Source: CAD feature listing. Evaluate the final solid. Frame: model axes, mm. A direction names the side the tool comes from. Give positions to 0.01 mm unless a question says otherwise; leave off trailing zeros. Loops run counter-clockwise (first coordinate to the right, second up) from the corner with the lowest first, then second, coordinate; pieces in that order, holes last.
```python
from build123d import *

# Parameters (mm, degrees)
SKETCH_1_W          = 30
SKETCH_1_H          = 36
SKETCH_1_R          = 1.7
EXTRUDE_1_DEPTH     = 8
SKETCH_2_R          = 3.75
CUT_EXTRUDE_1_DEPTH = 4.5
SKETCH_3_W          = 15
SKETCH_3_H          = 20
SKETCH_3_R          = 4
EXTRUDE_4_DEPTH     = 8
SKETCH_8_W          = 10
SKETCH_8_H          = 40
EXTRUDE_5_DEPTH     = 30
SKETCH_10_W         = 12
SKETCH_10_H         = 12.5
SKETCH_10_W_2       = 5
CUT_EXTRUDE_4_DEPTH = 30
SKETCH_11_R         = 1.5
CUT_EXTRUDE_5_DEPTH = 47
SKETCH_12_W         = 2
SKETCH_12_H         = 25.842259392
SKETCH_12_H_2       = 30.756424204
CUT_EXTRUDE_6_DEPTH = 10
SKETCH_13_R         = 1.5
CUT_EXTRUDE_7_DEPTH = 40
SKETCH_14_W         = 5
SKETCH_14_H         = 12.5
CUT_EXTRUDE_8_DEPTH = 10


with BuildPart() as part:
    # 草图1 → 凸台-拉伸1 (new body)
    with BuildSketch(Plane.XY):
        with Locations((-3.375, -1.625)):
            Rectangle(SKETCH_1_W, SKETCH_1_H)
        with Locations((-12.375, 10.375)):
            Circle(SKETCH_1_R, mode=Mode.SUBTRACT)
        with Locations((-12.375, -13.625)):
            Circle(SKETCH_1_R, mode=Mode.SUBTRACT)
        with Locations(Location((5.625, -13.625, 0), (0, 0, 180))):
            Circle(SKETCH_1_R, mode=Mode.SUBTRACT)
        with Locations(Location((5.625, 10.375, 0), (0, 0, 180))):
            Circle(SKETCH_1_R, mode=Mode.SUBTRACT)
    extrude(amount=EXTRUDE_1_DEPTH)

    # 草图2 → 切除-拉伸1 (cut)
    with BuildSketch(Plane(origin=(0, 0, 0), x_dir=(-1, 0, 0), z_dir=(0, 0, -1))):
        with Locations((12.375, 10.375)):
            Circle(SKETCH_2_R)
        with Locations(Location((-5.625, 10.375, 0), (0, 0, 180))):
            Circle(SKETCH_2_R)
        with Locations(Location((12.375, -13.625, 0), (0, 0, 180))):
            Circle(SKETCH_2_R)
        with Locations((-5.625, -13.625)):
            Circle(SKETCH_2_R)
    extrude(amount=-CUT_EXTRUDE_1_DEPTH, mode=Mode.SUBTRACT)

    # 草图3 → 凸台-拉伸4 (add)
    # profile 1 of 2: a face of its own
    with BuildSketch(Plane.XY.offset(8)):
        with Locations((-10.875, 26.375)):
            Rectangle(SKETCH_3_W, SKETCH_3_H)
        with Locations((-10.875, 21.375)):
            Circle(SKETCH_3_R, mode=Mode.SUBTRACT)
    # profile 2 of 2: a face of its own
    with BuildSketch(Plane.XY.offset(8)):
        with Locations((-10.875, -29.625)):
            Rectangle(SKETCH_3_W, SKETCH_3_H)
        with Locations((-10.875, -24.625)):
            Circle(SKETCH_3_R, mode=Mode.SUBTRACT)
    extrude(amount=-EXTRUDE_4_DEPTH)

    # 草图8 → 凸台-拉伸5 (add)
    with BuildSketch(Plane.XY.offset(8)):
        with Locations((16.625, -1.625)):
            Rectangle(SKETCH_8_W, SKETCH_8_H)
    extrude(amount=-EXTRUDE_5_DEPTH)

    # 草图10 → 切除-拉伸4 (cut)
    with BuildSketch(Plane.ZY.offset(-11.625)):
        with Locations((-16, 7.125)):
            Rectangle(SKETCH_10_W, SKETCH_10_H)
        with Locations((-2.5, 7.125)):
            Rectangle(SKETCH_10_W_2, SKETCH_10_H)
        with Locations((-2.5, -10.375)):
            Rectangle(SKETCH_10_W_2, SKETCH_10_H)
        with Locations((-16, -10.375)):
            Rectangle(SKETCH_10_W, SKETCH_10_H)
    extrude(amount=-CUT_EXTRUDE_4_DEPTH, mode=Mode.SUBTRACT)

    # 草图11 → 切除-拉伸5 (cut)
    with BuildSketch(Plane(origin=(0, 18.375, 0), x_dir=(1, 0, 0), z_dir=(0, 1, 0))):
        with Locations(Location((16.621809271, 18.123313308, 0), (0, 0, 180))):
            Circle(SKETCH_11_R)
    extrude(amount=-CUT_EXTRUDE_5_DEPTH, mode=Mode.SUBTRACT)

    # 草图12 → 切除-拉伸6 (cut)
    with BuildSketch(Plane(origin=(0, 0, 0), x_dir=(-1, 0, 0), z_dir=(0, 0, -1))):
        with Locations((10.875, 36.375)):
            Rectangle(SKETCH_12_W, SKETCH_12_H)
        with Locations((10.875, -39.625)):
            Rectangle(SKETCH_12_W, SKETCH_12_H_2)
    extrude(amount=-CUT_EXTRUDE_6_DEPTH, mode=Mode.SUBTRACT)

    # 草图13 → 切除-拉伸7 (cut)
    with BuildSketch(Plane.ZY.offset(18.375)):
        with Locations((3.892451488, 31.868119268)):
            Circle(SKETCH_13_R)
        with Locations(Location((3.892451488, -35.118119268, 0), (0, 0, 270))):
            Circle(SKETCH_13_R)
    extrude(amount=-CUT_EXTRUDE_7_DEPTH, mode=Mode.SUBTRACT)

    # 草图14 → 切除-拉伸8 (cut)
    with BuildSketch(Plane(origin=(21.625, 0, 0), x_dir=(0, 0, -1), z_dir=(1, 0, 0))):
        with Locations((7.5, 7.125)):
            Rectangle(SKETCH_14_W, SKETCH_14_H)
        with Locations((7.5, -10.375)):
            Rectangle(SKETCH_14_W, SKETCH_14_H)
    extrude(amount=-CUT_EXTRUDE_8_DEPTH, mode=Mode.SUBTRACT)


solid = part.part
```
(1) Section A-A, the plane z = -12.5. Return the cut outline in (x, y) (3 decimals).
A:
outline: (11.625, -21.625) - (21.625, -21.625) - (21.625, -16.625) - (11.625, -16.625) - close; (11.625, -4.125) - (21.625, -4.125) - (21.625, 0.875) - (11.625, 0.875) - close; (11.625, 13.375) - (21.625, 13.375) - (21.625, 18.375) - (11.625, 18.375) - close
(2) Section C-C, the plane x = 14. Return the cut outline in (y, z) (3 decimals).
A:
outline: (-21.625, -22) - (-16.625, -22) - (-16.625, 0) - (-4.125, 0) - (-4.125, -22) - (0.875, -22) - (0.875, 0) - (13.375, 0) - (13.375, -22) - (18.375, -22) - (18.375, 8) - (-21.625, 8) - close
(3) Ray query, line 1 along Y through (x, z) = (18.5, -13.25) (3 decimals); line 2 along X through (y, z) = (12, 3.5) (3 decimals); line 3 along Y through (x, z) = (20, 2) (3 decimals). Return the intervals inside material, ascending.
A:
line 1: y = -21.625 to -16.625, -4.125 to 0.875, 13.375 to 18.375
line 2: x = -18.375 to -15.755, -8.995 to 2.245, 9.005 to 21.625
line 3: y = -21.625 to 18.375
(4) Reachability of faces 5 (the flat face through (-18.375, -2, 4)), 6 (the cylindrical face through (18.12, -19.09, -18.06)), 7 (the flat face through (17, 13.375, -11)), 8 (the flat face through (17, 18.375, -7)), 9 (the flat face through (-9.875, 29, 4)) from +Z, -Z, +X, -X, +Y, -Y: full face, straight path, thin tool, end or side. Return the list, or none.
A:
face 5: +Z, -Z, -X, +Y, -Y
face 6: +Y, -Y
face 7: -Z, +X, -X
face 8: +Z, -Z, +X, +Y
face 9: +Z, -Z, +Y
(5) First-contact query: pin 1 (2 mm diameter, centred on x = 4.5, y = -15, fed in from -Z); pin 2 (11 mm diameter, centred on x = 18.5, z = -15, fed in from +Y) (3 decimals); pin 3 (4 mm diameter, centred on y = -35, z = 2.5, fed in from +X) (3 decimals). Flat tips, straight axial feed; report the tip coordinate or a pass-through.
A:
pin 1: stops at z = 4.5
pin 2: stops at y = 18.375
pin 3: stops at x = -3.375
(6) Section B-B, the plane y = -32. Return the cut outline in (x, z) (3 decimals).
A:
outline: (-18.375, 0) - (-11.875, 0) - (-11.875, 8) - (-18.375, 8) - close; (-9.875, 0) - (-3.375, 0) - (-3.375, 8) - (-9.875, 8) - close
(7) Section D-D, the plane y = 0. Return the cut outline in (x, z) (3 decimals).
A:
outline: (-18.375, 0) - (11.625, 0) - (11.625, -22) - (21.625, -22) - (21.625, 8) - (-18.375, 8) - close; hole circle Ø3 at (16.622, -18.123)
(8) Mould query, pull axis Z, two halves, no side actions, for faces 1 (the flat face through (17, 0.875, -11)), 2 (the cylindrical face through (-6.671, 30.404, 3.567)), 3 (the flat face through (-3, -1, 8)), 4 (the flat face through (7, 9, 4.5)). Classes: pulls with the +Z half, pulls with the -Z half, needs draft (parallel to the pull), parting line crosses it, or undercut.
A:
face 1: needs draft
face 2: undercut
face 3: pulls with the +Z half
face 4: pulls with the -Z half
